```python
from build123d import *

# Parameters (mm, degrees)
BOSS_EXTRUDE1_DEPTH      = 40
BOSS_EXTRUDE1_DEPTH_BACK = 40
SKETCH1_R                = 20
CUT_EXTRUDE1_DEPTH       = 4.9
SKETCH3_R                = 22.5
BOSS_EXTRUDE2_DEPTH      = 21
SKETCH4_R                = 17.5
BOSS_EXTRUDE3_DEPTH      = 18
CHAMFER1_SIZE            = 1
BOSS_EXTRUDE4_START      = 100
SKETCH5_R                = 17.5
BOSS_EXTRUDE4_DEPTH      = 100
SKETCH6_R                = 17
BOSS_EXTRUDE5_DEPTH      = 60
CUT_EXTRUDE2_DEPTH       = 4.1
CHAMFER2_SIZE            = 1


with BuildPart() as part:
    # Sketch1 → Boss-Extrude1 (new, two sides: drawn at the far end of the back side and taken through both)
    with BuildSketch(Plane(origin=(0, 0, 0), x_dir=(0, 0, -1), z_dir=(1, 0, 0)).offset(-BOSS_EXTRUDE1_DEPTH_BACK)):
        Circle(SKETCH1_R)
    extrude(amount=BOSS_EXTRUDE1_DEPTH + BOSS_EXTRUDE1_DEPTH_BACK)

    # Sketch2 → Cut-Extrude1 (cut)
    with BuildSketch(Plane(origin=(0, 20, 0), x_dir=(1, 0, 0), z_dir=(0, 1, 0))):
        with BuildLine():
            Line((-19, 6), (19, 6))
            ThreePointArc((19, 6), (25, 0), (19, -6))
            Line((19, -6), (-19, -6))
            ThreePointArc((-19, -6), (-25, 0), (-19, 6))
        make_face()
    extrude(amount=-CUT_EXTRUDE1_DEPTH, mode=Mode.SUBTRACT)

    # Sketch3 → Boss-Extrude2 (add)
    with BuildSketch(Plane.ZY.offset(40)):
        with Locations(Location((0, 0, 0), (0, 0, 180))):
            Circle(SKETCH3_R)
    extrude(amount=BOSS_EXTRUDE2_DEPTH)

    # Sketch4 → Boss-Extrude3 (add)
    with BuildSketch(Plane.ZY.offset(61)):
        Circle(SKETCH4_R)
    extrude(amount=BOSS_EXTRUDE3_DEPTH)

    # Chamfer1
    chamfer1_edges = [part.edges().sort_by_distance(p)[0] for p in [
        (-79, 0, -17.5),
    ]]
    chamfer(chamfer1_edges, length=CHAMFER1_SIZE)

    # Sketch5 → Boss-Extrude4 (add)
    with BuildSketch(Plane(origin=(40, 0, 0), x_dir=(0, 0, -1), z_dir=(1, 0, 0)).offset(BOSS_EXTRUDE4_START)):
        with Locations(Location((0, 0, 0), (0, 0, 180))):
            Circle(SKETCH5_R)
    extrude(amount=-BOSS_EXTRUDE4_DEPTH)

    # Sketch6 → Boss-Extrude5 (add)
    with BuildSketch(Plane(origin=(140, 0, 0), x_dir=(0, 0, -1), z_dir=(1, 0, 0))):
        Circle(SKETCH6_R)
    extrude(amount=BOSS_EXTRUDE5_DEPTH)

    # Sketch7 → Cut-Extrude2 (cut)
    with BuildSketch(Plane(origin=(0, 17, 0), x_dir=(1, 0, 0), z_dir=(0, 1, 0))):
        with BuildLine():
            Line((152, 5), (188, 5))
            ThreePointArc((188, 5), (193, 0), (188, -5))
            Line((188, -5), (152, -5))
            ThreePointArc((152, -5), (147, 0), (152, 5))
        make_face()
    extrude(amount=-CUT_EXTRUDE2_DEPTH, mode=Mode.SUBTRACT)

    # Chamfer2
    chamfer2_edges = [part.edges().sort_by_distance(p)[0] for p in [
        (200, 0, 17),
    ]]
    chamfer(chamfer2_edges, length=CHAMFER2_SIZE)


solid = part.part
```
Part model, mm, in its own coordinate system. A direction names the side the tool comes from. Round coordinates to 2 decimals unless told otherwise and drop trailing zeros. Write each loop counter-clockwise with the first axis right and the second up, starting at its lowest first coordinate (ties: lowest second). Pieces come first, ordered by that corner, then holes. Notation, with made-up numbers: M 3,82 L 15,82 A31 cw 15,106 Z; hole C 11.25,26.5 d4. An arc over 180 degrees is marked long. Answer as CSV lines item,"result". Start each with the question number.
1) Which spindle directions (+Z, -Z, +X, -X, +Y, -Y) get a long thin tool onto all of the face, cutting with end or side? Do faces 1 (the face through (-0.56, -19.524, 4.336)), 2 (the face through (193, 15, 0)), 3 (the face through (-79, 0, 0)). Say none if no direction does.
2) Band-saw the part on A-A (x = 130). List the corners of the cut face in (y, z).
3) Drill centre lines: L1, parallel to Y at x = 52, z = 1; L2, parallel to Y at x = 178, z = 0; L3, parallel to X at y = 6.5, z = 16.5. Where is each one in solid material? Low to high.
4) Mould opens along Z. For faces 4 (the face through (-25, 18, 0)), 5 (the face through (-69.381, -10.648, -13.887)), 6 (the face through (147, 15, 0)), 7 (the face through (-61, 13, -12)) say: +Z half, -Z half, draft (parallel to the pull), parting line (faces both ways), or undercut.
5) Drop flat-ended pins along their axis: pin 1 (1 mm diameter, centred on x = 163.5, y = 14, fed in from -Z); pin 2 (1 mm diameter, centred on x = 18.5, z = 10, fed in from -Y); pin 3 (10 mm diameter, centred on x = 89.5, y = -16.5, fed in from -Z). Give the stop position or say it passes through.
Worked out:
1,face 1,"+X"
1,face 2,"+Y"
1,face 3,"+Z, -Z, -X, +Y, -Y"
2,outline,"C 0,0 d35"
3,L1,"-17.47 to 17.47"
3,L2,"-17 to 12.9"
3,L3,"-61 to 40"
4,face 4,"undercut"
4,face 5,"parting line"
4,face 6,"undercut"
4,face 7,"draft"
5,pin 1,"z = -10.33"
5,pin 2,"y = -17.6"
5,pin 3,"z = -13.19"
